```python
from build123d import *

# Parameters (mm, degrees)
SKETCH1_W           = 4
SKETCH1_H           = 10
SKETCH1_H_2         = 30.5
SKETCH1_W_2         = 34.5
SKETCH1_H_3         = 4
SKETCH1_W_3         = 26.5
SKETCH1_W_4         = 10
BOSS_EXTRUDE1_DEPTH = 42
CUT_EXTRUDE1_DEPTH  = 34
SKETCH3_R           = 1.75
CUT_EXTRUDE2_DEPTH  = 72.529714105
SKETCH3_3_R         = 1.75
CUT_EXTRUDE3_DEPTH  = 2
SKETCH4_R           = 1.75
CUT_EXTRUDE4_DEPTH  = 72.249561402
SKETCH4_3_R         = 1.75
CUT_EXTRUDE5_DEPTH  = 2
SKETCH5_R           = 1.75
CUT_EXTRUDE6_DEPTH  = 72.249561402
SKETCH5_3_R         = 1.75
CUT_EXTRUDE7_DEPTH  = 2
FILLET1_R           = 10


with BuildPart() as part:
    # Sketch1 → Boss-Extrude1 (new body)
    with BuildSketch(Plane.XY):
        Polygon((8, 8), (34.5, 8), (44.5, 8), (44.5, 44.5), (8, 44.5), (8, 34.5), align=None)
        with Locations((6, 39.5)):
            Rectangle(SKETCH1_W, SKETCH1_H)
        with Locations((2, 39.5)):
            Rectangle(SKETCH1_W, SKETCH1_H)
        with Locations((2, 19.25)):
            Rectangle(SKETCH1_W, SKETCH1_H_2)
        Polygon((4, 34.5), (4, 4), (8, 4), (8, 8), (8, 34.5), align=None)
        with Locations((17.25, 2)):
            Rectangle(SKETCH1_W_2, SKETCH1_H_3)
        with Locations((21.25, 6)):
            Rectangle(SKETCH1_W_3, SKETCH1_H_3)
        with Locations((39.5, 6)):
            Rectangle(SKETCH1_W_4, SKETCH1_H_3)
        with Locations((39.5, 2)):
            Rectangle(SKETCH1_W_4, SKETCH1_H_3)
    extrude(amount=BOSS_EXTRUDE1_DEPTH)

    # Sketch1<3> → Cut-Extrude1 (cut)
    with BuildSketch(Plane.XY):
        Polygon((8, 8), (34.5, 8), (44.5, 8), (44.5, 44.5), (8, 44.5), (8, 34.5), align=None)
    extrude(amount=CUT_EXTRUDE1_DEPTH, mode=Mode.SUBTRACT)

    # Sketch3 → Cut-Extrude2 (cut, through all)
    with BuildSketch(Plane(origin=(0, 0, 34), x_dir=(-1, 0, 0), z_dir=(0, 0, -1))):
        with Locations((-34.5, 34.5)):
            Circle(SKETCH3_R)
    extrude(amount=-CUT_EXTRUDE2_DEPTH, mode=Mode.SUBTRACT)

    # Sketch3<3> → Cut-Extrude3 (cut)
    with BuildSketch(Plane(origin=(0, 0, 34), x_dir=(-1, 0, 0), z_dir=(0, 0, -1))):
        Polygon((-31.266838493, 34.5), (-32.883419246, 37.3), (-36.116580754, 37.3), (-37.733161507, 34.5), (-36.116580754, 31.7), (-32.883419246, 31.7), align=None)
        with Locations((-34.5, 34.5)):
            Circle(SKETCH3_3_R, mode=Mode.SUBTRACT)
    extrude(amount=-CUT_EXTRUDE3_DEPTH, mode=Mode.SUBTRACT)

    # Sketch4 → Cut-Extrude4 (cut, through all)
    with BuildSketch(Plane(origin=(8, 0, 0), x_dir=(0, 0, -1), z_dir=(1, 0, 0))):
        with Locations(Location((-10, 34.5, 0), (0, 0, 90))):
            Circle(SKETCH4_R)
    extrude(amount=-CUT_EXTRUDE4_DEPTH, mode=Mode.SUBTRACT)

    # Sketch4<3> → Cut-Extrude5 (cut)
    with BuildSketch(Plane(origin=(8, 0, 0), x_dir=(0, 0, -1), z_dir=(1, 0, 0))):
        Polygon((-6.766838493, 34.5), (-8.383419246, 37.3), (-11.616580754, 37.3), (-13.233161507, 34.5), (-11.616580754, 31.7), (-8.383419246, 31.7), align=None)
        with Locations(Location((-10, 34.5, 0), (0, 0, 90))):
            Circle(SKETCH4_3_R, mode=Mode.SUBTRACT)
    extrude(amount=-CUT_EXTRUDE5_DEPTH, mode=Mode.SUBTRACT)

    # Sketch5 → Cut-Extrude6 (cut, through all)
    with BuildSketch(Plane(origin=(0, 8, 0), x_dir=(1, 0, 0), z_dir=(0, 1, 0))):
        with Locations(Location((34.5, -10, 0), (0, 0, 270))):
            Circle(SKETCH5_R)
    extrude(amount=-CUT_EXTRUDE6_DEPTH, mode=Mode.SUBTRACT)

    # Sketch5<3> → Cut-Extrude7 (cut)
    with BuildSketch(Plane(origin=(0, 8, 0), x_dir=(1, 0, 0), z_dir=(0, 1, 0))):
        Polygon((37.733161507, -10), (36.116580754, -7.2), (32.883419246, -7.2), (31.266838493, -10), (32.883419246, -12.8), (36.116580754, -12.8), align=None)
        with Locations(Location((34.5, -10, 0), (0, 0, 270))):
            Circle(SKETCH5_3_R, mode=Mode.SUBTRACT)
    extrude(amount=-CUT_EXTRUDE7_DEPTH, mode=Mode.SUBTRACT)

    # Fillet1
    fillet1_edges = [part.edges().sort_by_distance(p)[0] for p in [
        (44.5, 44.5, 38),
        (0, 0, 21),
        (0, 22.25, 42),
        (44.5, 4, 0),
        (22.25, 0, 42),
        (8, 8, 17),
        (8, 26.25, 34),
        (26.25, 8, 34),
        (4, 44.5, 0),
    ]]
    fillet(fillet1_edges, radius=FILLET1_R)


solid = part.part
```
Input: part model. Units: mm. Frame: model coordinates. A direction names the side the tool comes from. Coordinates: 2 decimals unless noted, no trailing zeros. Order: outer loops, then holes, each group sorted by start corner. A loop starts at its lowest first (then second) coordinate and runs counter-clockwise, first axis right, second up. Notation, with made-up numbers: (31, 48.25) - (35, 48.25) arc R32 cw to (35, 75.25) - close; hole circle Ø11 at (21, 72). An arc over 180 degrees is marked (long way). Return JSON: item names as keys, results as strings.
Q1. Draft query along X for faces 1 (the cylindrical face through (41.49, 4.06, 2.85)), 2 (the flat face through (7, 37.3, 10)), 3 (the flat face through (34, 37.3, 35)). Return one class per face: +X half, -X half, draft (parallel to the pull), parting line (faces both ways), or undercut.
The answers:
{"face 1": "+X half", "face 2": "draft", "face 3": "undercut"}
Q2. Cut plane D-D (z = 37.5). Return loops of the section in (x, y), then the cut area to 3 significant figures.
The answers:
{"outline": "(1.65, 10) arc R8.35 ccw to (10, 1.65) - (44.5, 1.65) - (44.5, 34.5) arc R10 ccw to (34.5, 44.5) - (1.65, 44.5) - close; hole circle Ø3.5 at (34.5, 34.5)", "area": "1,790 mm2"}
Q3. Cut plane A-A (x = 4). Return loops of the section in (y, z), then the cut area to 3 significant figures.
The answers:
{"outline": "(2, 0) - (34.5, 0) arc R10 ccw to (44.5, 10) - (44.5, 40) - (10, 40) arc R8 ccw to (2, 32) - close; hole circle Ø3.5 at (34.5, 10)", "area": "1,660 mm2"}
Q4. Ray query, probe 1 along Y at (x, z) = (12, 10.5); probe 2 along Y at (x, z) = (34.5, 38.4); probe 3 along Z at (x, y) = (41.5, 24.5). Return the intervals inside material, ascending.
The answers:
{"probe 1": "y = 0 to 10", "probe 2": "y = 2.32 to 32.75, 36.25 to 44.5", "probe 3": "z = 34 to 42"}
Q5. Cut plane B-B (y = 26). Return loops of the section in (x, z), then the cut area to 3 significant figures.
The answers:
{"outline": "(0, 0) - (8, 0) - (8, 24) arc R10 cw to (18, 34) - (44.5, 34) - (44.5, 42) - (10, 42) arc R10 ccw to (0, 32) - close", "area": "628 mm2"}
Q6. First-contact query: pin 1 (7 mm diameter, centred on x = 36, z = 15, fed in from +Y); pin 2 (5.5 mm diameter, centred on x = 34.5, y = 34.5, fed in from +Z); pin 3 (4.5 mm diameter, centred on x = 34.5, z = 10, fed in from +Y); pin 4 (3 mm diameter, centred on y = 19.5, z = 23.5, fed in from +X). Flat tips, straight axial feed; report the tip coordinate or a pass-through.
The answers:
{"pin 1": "stops at y = 8", "pin 2": "stops at z = 42", "pin 3": "stops at y = 6", "pin 4": "stops at x = 8.05"}
Q7. Access query for faces 4 (the flat face through (32.086, 7.014, 8.58)), 5 (the flat face through (33, 33, 36)), 6 (the flat face through (7.014, 35.88, 7.564)). Directions: +Z, -Z, +X, -X, +Y, -Y. A direction counts if a zero-diameter tool reaches every point of the face in a straight line with its end or side. Return the directions, or none.
The answers:
{"face 4": "+Y", "face 5": "-Z", "face 6": "+X"}
